Could you check a few things on this model? Use its own coordinates, in mm. A direction names the side the tool comes from. Give positions to 0.01 mm unless a question says otherwise; leave off trailing zeros. Write each question's results on one line, items separated by ' | '. Start each with the question number.
(1) On a 3-axis mill with a long thin cutter (end or side, diameter ignored), from which of +Z, -Z, +X, -X, +Y, -Y can I reach the whole of each face in a straight line? I mean faces 1 (the face through (59, 0, -4.95)), 2 (the face through (5.5, 0, 3)), 3 (the face through (114.5, 0, 3)), 4 (the face through (3, 0, -1.95)), 5 (the face through (114.5, 0, -3)). Say none if no direction works.
(2) Suppose I cut it at A-A (y = 0). Count the separate pieces of the cut face and the enclosed holes in it, and give its area (3 significant figures).
(3) If we mould it in two halves opening along Y, with no side actions, what happens to faces 6 (the face through (59, 5, 0)), 7 (the face through (-4.634, -0.102, 1.815)), 8 (the face through (121.526, 0.481, -0.02))? For each: released by +Y, released by -Y, zero draft, split by the parting line, or undercut.
(4) I need wall thicknesses on line 1 (Y direction, x = 0, z = -0.7); line 2 (X direction, y = -1, z = 1); line 3 (X direction, y = -0.5, z = 2.5). Which ranges of each line are inside material? Lowest first, please.
(5) For pin 1 (4.5 mm diameter, centred on x = 1, y = 0, fed in from -Z); pin 2 (4.5 mm diameter, centred on x = 121, y = 1.5, fed in from +Z); pin 3 (2 mm diameter, centred on y = 1.5, z = 3, fed in from +X); pin 4 (3 mm diameter, centred on x = 120, y = 0, fed in from +Z), each with a flat end and sliding along its axis, tell me the tip position at first contact or that it passes through.
from build123d import *

# Parameters (mm, degrees)
BOSS_EXTRUDE1_DEPTH      = 1.95
BOSS_EXTRUDE1_DEPTH_BACK = 1.95
SKETCH1_R                = 1.6
BOSS_EXTRUDE2_DEPTH      = 3.1
BOSS_EXTRUDE2_DEPTH_BACK = 6.9
SKETCH2_W                = 109
SKETCH2_H                = 10
CHAMFER1_SIZE            = 0.5


with BuildPart() as part:
    # Sketch1 → Boss-Extrude1 (new, two sides: drawn at the far end of the back side and taken through both)
    with BuildSketch(Plane.XY.offset(-BOSS_EXTRUDE1_DEPTH_BACK)):
        with BuildLine():
            Line((0, 5), (120, 5))
            ThreePointArc((120, 5), (125, 0), (120, -5))
            Line((120, -5), (0, -5))
            ThreePointArc((0, -5), (-5, 0), (0, 5))
        make_face()
        Circle(SKETCH1_R, mode=Mode.SUBTRACT)
        with Locations((120, 0)):
            Circle(SKETCH1_R, mode=Mode.SUBTRACT)
    extrude(amount=BOSS_EXTRUDE1_DEPTH + BOSS_EXTRUDE1_DEPTH_BACK)

    # Sketch2 → Boss-Extrude2 (add, two sides: drawn at the far end of the back side and taken through both)
    with BuildSketch(Plane.XY.offset(1.95).offset(-BOSS_EXTRUDE2_DEPTH_BACK)):
        with Locations((60, 0)):
            Rectangle(SKETCH2_W, SKETCH2_H)
    extrude(amount=BOSS_EXTRUDE2_DEPTH + BOSS_EXTRUDE2_DEPTH_BACK)

    # Chamfer1
    chamfer1_edges = [part.edges().sort_by_distance(p)[0] for p in [
        (125, 0, -1.95),
        (-1.6, 0, -1.95),
        (117.25, 5, -1.95),
        (118.4, 0, -1.95),
        (-5, 0, 1.95),
        (2.75, -5, 1.95),
        (125, 0, 1.95),
        (117.25, 5, 1.95),
        (-1.6, 0, 1.95),
        (118.4, 0, 1.95),
        (117.25, -5, 1.95),
        (2.75, 5, 1.95),
        (2.75, 5, -1.95),
        (117.25, -5, -1.95),
        (-5, 0, -1.95),
        (5.5, 0, -4.95),
        (5.5, -5, -3.45),
        (60, 5, -4.95),
        (5.5, 5, -3.45),
        (114.5, 0, -4.95),
        (114.5, 5, -3.45),
        (60, -5, -4.95),
        (114.5, -5, -3.45),
        (5.5, -5, 3.5),
        (5.5, 5, 3.5),
        (114.5, 5, 3.5),
        (114.5, -5, 3.5),
        (5.5, 0, 5.05),
        (60, -5, 5.05),
        (114.5, 0, 5.05),
        (60, 5, 5.05),
        (2.75, -5, -1.95),
    ]]
    chamfer(chamfer1_edges, length=CHAMFER1_SIZE)


solid = part.part
Output values:
1) face 1: -Z, +X, -X, +Y, -Y | face 2: +Z, -X, +Y, -Y | face 3: +Z, +X, +Y, -Y | face 4: -Z, -X, +Y, -Y | face 5: -Z, +X, +Y, -Y
2) separate pieces: 3 | enclosed holes: 0 | area: 1,140 mm2
3) face 6: released by +Y | face 7: split by the parting line | face 8: undercut
4) line 1: -5 to -1.6, 1.6 to 5 | line 2: -4.9 to -1.25, 1.25 to 118.75, 121.25 to 124.9 | line 3: 5.5 to 114.5
5) pin 1: z = -1.95 | pin 2: z = 1.95 | pin 3: x = 114.5 | pin 4: through
